Verification items for the finished model (mm, model axes). Face numbers are marked on the shaded views. Give positions to 0.01 mm unless a question says otherwise; leave off trailing zeros. Order: outer loops, then holes, each group sorted by start corner. A loop starts at its lowest first (then second) coordinate and runs counter-clockwise, first axis right, second up.
(1) Gauge pin test, flat end, axial feed: pin 1 (2 mm diameter, centred on y = 4, z = -4.5, fed in from -X). Record the tip position at first contact, or that the pin passes through.
(2) Mould release check, pull along X, two halves, no side actions. Record for the marked faces 1, 2 and 3: pulls with the +X half, pulls with the -X half, needs draft (parallel to the pull), parting line crosses it, or undercut.
(3) Scan lines: L1, parallel to X at y = 4.5, z = -5; L2, parallel to Y at x = 20, z = -7.5 (3 decimals); L3, parallel to X at y = 6, z = -8. Record each from-to range of solid material in increasing order.
(4) Sectioned sample at B-B on x = 20. Record the cut outline in (y, z) (3 decimals).
(5) Sectioned sample at A-A on z = -5. Record the cut outline in (x, y) (3 decimals).
(6) Sectioned sample at D-D on y = 8.5. Record the cut outline in (x, z).
(7) Sectioned sample at C-C on y = 6.25. Record the cut outline in (x, z).
```python
from build123d import *

# Parameters (mm, degrees)
SKETCH1_W             = 40
SKETCH1_H             = 10
BOSS_EXTRUDE1_DEPTH   = 11.65
M3X0_5_TAPPED_HOLE3_D = 2.5
M3X0_5_TAPPED_HOLE4_D = 2.5


with BuildPart() as part:
    # Sketch1 → Boss-Extrude1 (new body)
    with BuildSketch(Plane(origin=(0, 0, 0), x_dir=(1, 0, 0), z_dir=(0, 1, 0))):
        with Locations((20, 5)):
            Rectangle(SKETCH1_W, SKETCH1_H)
    extrude(amount=BOSS_EXTRUDE1_DEPTH)

    # M3x0.5 Tapped Hole3 (through all)
    with Locations(Plane(origin=(5, 11.65, -5), x_dir=(0, 0, 1), z_dir=(0, 1, 0))):
        with Locations((0, 0), (0, 30)):
            Hole(M3X0_5_TAPPED_HOLE3_D / 2)

    # M3x0.5 Tapped Hole4 (through all)
    with Locations(Plane(origin=(20, 5.825, -10), x_dir=(-1, 0, 0), z_dir=(0, 0, -1))):
        with Locations((0, 0)):
            Hole(M3X0_5_TAPPED_HOLE4_D / 2)


solid = part.part
```
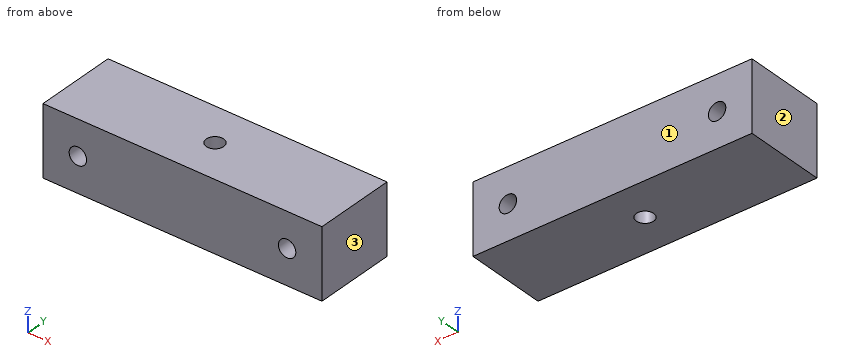
Ans:
1. pin 1: stops at x = 0
2. face 1: needs draft
2. face 2: pulls with the -X half
2. face 3: pulls with the +X half
3. L1: x = 0 to 3.75, 6.25 to 33.75, 36.25 to 40
3. L2: y = 0 to 4.575, 7.075 to 11.65
3. L3: x = 0 to 18.76, 21.24 to 40
4. outline: (0, -10) - (4.575, -10) - (4.575, 0) - (0, 0) - close; (7.075, -10) - (11.65, -10) - (11.65, 0) - (7.075, 0) - close
5. outline: (0, 0) - (3.75, 0) - (3.75, 11.65) - (0, 11.65) - close; (6.25, 0) - (33.75, 0) - (33.75, 11.65) - (6.25, 11.65) - close; (36.25, 0) - (40, 0) - (40, 11.65) - (36.25, 11.65) - close; hole circle Ø2.5 at (20, 5.825)
6. outline: (0, -10) - (40, -10) - (40, 0) - (0, 0) - close; hole circle Ø2.5 at (5, -5); hole circle Ø2.5 at (35, -5)
7. outline: (0, -10) - (18.82, -10) - (18.82, 0) - (0, 0) - close; (21.18, -10) - (40, -10) - (40, 0) - (21.18, 0) - close; hole circle Ø2.5 at (5, -5); hole circle Ø2.5 at (35, -5)
